Source: CAD feature listing. Evaluate the final solid. Frame: model axes, mm. Face numbers are marked on the shaded views. A direction names the side the tool comes from. Give positions to 0.01 mm unless a question says otherwise; leave off trailing zeros. Order: outer loops, then holes, each group sorted by start corner. A loop starts at its lowest first (then second) coordinate and runs counter-clockwise, first axis right, second up.
```python
from build123d import *

# Parameters (mm, degrees)
F0_W     = 1.5
F0_H     = 6.264
F2_DEPTH = 255
F3_SIZE2 = 0.7053079228
F3_SIZE  = 4


with BuildPart() as f1:
    # F0 (on Front) → F1 (revolve)
    with BuildSketch(Plane.XZ):
        with BuildLine():
            Line((-1.8977640684, 2.5627018091), (-0.8977640684, 2.5627018091))
            Line((-0.8977640684, 2.5627018091), (-0.8977640684, -18.4372981909))
            Line((-0.8977640684, -18.4372981909), (1.1022359316, -26.1832648833))
            Line((1.1022359316, -26.1832648833), (2.6022359316, -26.1832648833))
            Line((2.6022359316, -26.1832648833), (0.6253340279, -18.3980558312))
            Line((0.6253340279, -18.3980558312), (0.6022359316, 8.5731884591))
            Line((0.6022359316, 8.5731884591), (-1.8977640684, 8.5627018091))
            Line((-1.8977640684, 8.5627018091), (-1.8977640684, 18.240797309))
            Line((-1.8977640684, 18.240797309), (0.1022359316, 22.2902958969))
            Line((0.1022359316, 22.2902958969), (0.1022359316, 22.5522806174))
            Line((0.1022359316, 22.5522806174), (-1.8977640684, 22.5522806174))
            Line((-1.8977640684, 22.5522806174), (-1.8977640684, 20.5522806174))
            ThreePointArc((-1.8977640684, 20.5522806174), (-2.483550506, 19.138067055), (-3.8977640684, 18.5522806174))
            Line((-3.8977640684, 18.5522806174), (-5.8977640684, 18.5522806174))
            Line((-5.8977640684, 18.5522806174), (-5.3977640684, 6.5627018091))
            Line((-5.3977640684, 6.5627018091), (-0.8977640684, 6.5627018091))
            Line((-0.8977640684, 6.5627018091), (-0.8977640684, 4.5627018091))
            Line((-0.8977640684, 4.5627018091), (-1.8977640684, 4.5627018091))
            Line((-1.8977640684, 4.5627018091), (-1.8977640684, 2.5627018091))
        make_face()
        with Locations((1.8522359316, -29.3152648833)):
            Rectangle(F0_W, F0_H)
    revolve(axis=Axis((21.1022359316, 0, -25.8119600499), (0, 0, 1)))

    # F2 (add): a face of the model
    f2_faces = [f1.faces().sort_by_distance(p)[0] for p in [
        (40.5365505067, 0, -32.4472648833),
    ]]
    extrude(f2_faces, amount=F2_DEPTH)

    # F3
    f3_edges = [f1.edges().sort_by_distance(p)[0] for p in [
        (41.102236, 0, -287.447265),
    ]]
    chamfer(f3_edges, length=F3_SIZE, length2=F3_SIZE2)


solid = f1.part
```
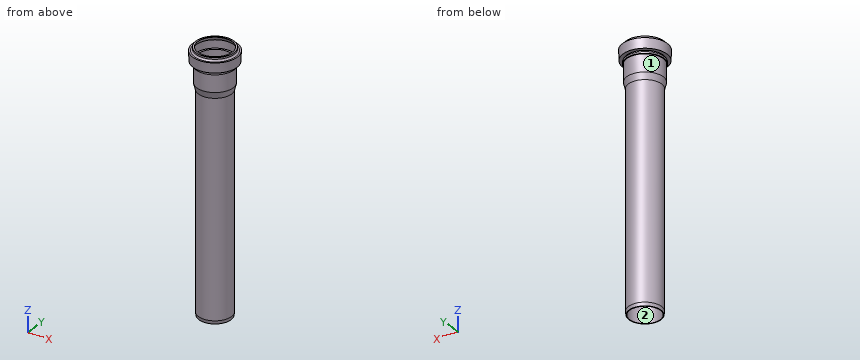
1) Pin query (flat end, axial travel): pin 1 (6 mm diameter, centred on x = 13, z = -35.5, fed in from -Y); pin 2 (8 mm diameter, centred on x = 0, y = -4.5, fed in from -Z); pin 3 (4 mm diameter, centred on x = 3.5, z = -49, fed in from -Y); pin 4 (3 mm diameter, centred on x = 20, z = -254, fed in from -Y). Return the tip coordinate at first contact, or that it passes through.
Report:
pin 1: stops at y = -19.34
pin 2: stops at z = -287.45
pin 3: stops at y = -12.51
pin 4: stops at y = -20
2) Material intervals for L1, parallel to X at y = 0, z = -107; L2, parallel to Z at x = 9.5, y = -19; L3, parallel to Z at x = 39, y = -19, sorted ascending.
Report:
L1: x = 1.1 to 2.6, 39.6 to 41.1
L2: z = 2.56 to 4.56, 6.56 to 8.57, 19.73 to 22.55
L3: z = 6.56 to 18.55
3) Section query A-A, the plane z = -229. Return the cut outline in (x, y).
Report:
outline: circle Ø40 at (21.1, 0); hole circle Ø37 at (21.1, 0)
4) Reachability of the marked faces 1 and 2 from +Z, -Z, +X, -X, +Y, -Y: full face, straight path, thin tool, end or side. Return the list, or none.
Report:
face 1: -Z
face 2: +Z, -Z
5) Section query B-B, the plane z = -12.5. Return the cut outline in (x, y), and give its area (3 significant figures).
Report:
outline: circle Ø44 at (21.1, 0); hole circle Ø40.96 at (21.1, 0)
area: 203 mm2
